Check sheet for the modelled part. Datum: model origin and axes. Units: mm. Round coordinates to 2 decimals unless told otherwise and drop trailing zeros. Order: outer loops, then holes, each group sorted by start corner. A loop starts at its lowest first (then second) coordinate and runs counter-clockwise, first axis right, second up. Notation, with made-up numbers: (11.5, -24.75) -> (50.5, -24.75) arc R38 cw to (50.5, 14.25) -> close; hole circle Ø4 at (78, 17). An arc over 180 degrees is marked (long way). Answer in a Markdown table with one row per item.
from build123d import *

# Parameters (mm, degrees)
F0_W     = 300
F0_H     = 100
F1_DEPTH = 20
F2_W     = 20
F2_H     = 20
F3_DEPTH = 20
F4_W     = 280
F4_H     = 10
F5_DEPTH = 10


with BuildPart() as f1:
    # F0 (on Right) → F1 (new body)
    with BuildSketch(Plane.YZ):
        Rectangle(F0_W, F0_H)
    extrude(amount=F1_DEPTH)

    # F2 (on face) → F3 (cut, through all)
    with BuildSketch(Plane(origin=(0, 0, 0), x_dir=(0, -1, 0), z_dir=(-1, 0, 0))):
        with Locations((140, -20)):
            Rectangle(F2_W, F2_H)
        with Locations((-140, -20)):
            Rectangle(F2_W, F2_H)
        with Locations((140, 20)):
            Rectangle(F2_W, F2_H)
        with Locations((-140, 20)):
            Rectangle(F2_W, F2_H)
    extrude(amount=-F3_DEPTH, mode=Mode.SUBTRACT)

    # F4 (on face) → F5 (cut)
    with BuildSketch(Plane.YZ.offset(20)):
        with Locations((0, 35)):
            Rectangle(F4_W, F4_H)
    extrude(amount=-F5_DEPTH, mode=Mode.SUBTRACT)


solid = f1.part
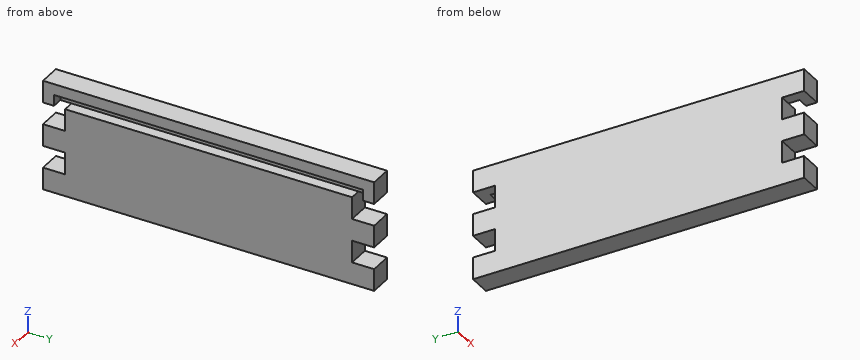
Item 1: Cross-section at D-D (z = -16). Record the boundary of the cut face in (x, y), and give its area (3 significant figures).
Result sheet:
| item | result |
|---|---|
| outline | (0, -130) -> (20, -130) -> (20, 130) -> (0, 130) -> close |
| area | 5,200 mm^2 |
Item 2: Cross-section at B-B (x = 3). Record the boundary of the cut face in (y, z).
Result sheet:
| item | result |
|---|---|
| outline | (-150, -50) -> (150, -50) -> (150, -30) -> (130, -30) -> (130, -10) -> (150, -10) -> (150, 10) -> (130, 10) -> (130, 30) -> (150, 30) -> (150, 50) -> (-150, 50) -> (-150, 30) -> (-130, 30) -> (-130, 10) -> (-150, 10) -> (-150, -10) -> (-130, -10) -> (-130, -30) -> (-150, -30) -> close |
Item 3: Cross-section at C-C (z = 37). Record the boundary of the cut face in (x, y).
Result sheet:
| item | result |
|---|---|
| outline | (0, -150) -> (20, -150) -> (20, -140) -> (10, -140) -> (10, 140) -> (20, 140) -> (20, 150) -> (0, 150) -> close |
Item 4: Depth check by flat-ended pin: P1, Ø5, axis at x = 12, z = 20.5, coming from the +Y side. Enter the tip coordinate at first touch or a pass-through.
Result sheet:
| item | result |
|---|---|
| P1 | stops at y = 130 |
Item 5: Cross-section at A-A (y = -92.5). Record the boundary of the cut face in (x, z).
Result sheet:
| item | result |
|---|---|
| outline | (0, -50) -> (20, -50) -> (20, 30) -> (10, 30) -> (10, 40) -> (20, 40) -> (20, 50) -> (0, 50) -> close |
Item 6: Scan lines: line 1 (Z direction, x = 11, y = 45); line 2 (Y direction, x = 16.5, z = 13.5); line 3 (X direction, y = -6.5, z = 32.5). Record each from-to range of solid material in increasing order. Write a range as [from, to].
Result sheet:
| item | result |
|---|---|
| line 1 | z = [-50, 30], [40, 50] |
| line 2 | y = [-130, 130] |
| line 3 | x = [0, 10] |
